```python
from build123d import *

# Parameters (mm, degrees)
F0_W          = 76.2
F0_H          = 38.1
F1_DEPTH      = 25.4
F2_W          = 69.85
F2_H          = 2.54
F3_DEPTH      = 38.101
F4_W          = 63.5
F4_H          = 25.4
F5_DEPTH      = 12.7
F6_W          = 6.35
F6_H          = 8.89
F7_DEPTH      = 6.35
F8_R          = 1.905
F9_DEPTH      = 6.35
F10_T1_DEPTH  = 76.2
F11_T1_DEPTH  = 17.78
F11_T3_DEPTH  = 55.88
F11_T5_DEPTH  = 7.62
F11_T7_DEPTH  = 7.62
F11_T10_ANGLE = 90.0000000017
F11_T12_ANGLE = 89.9999999998
F11_T14_ANGLE = 89.9999999979
F11_T16_ANGLE = 89.9999999998
F11_T18_ANGLE = 89.9999999998
F11_T20_ANGLE = 89.9999999998
F11_T22_ANGLE = 89.9999999979
F11_T24_ANGLE = 90.0000000017


# Not quite as in the source:
# - a fillet or chamfer that OpenCascade refuses, or shapes differently, is made with other operations: its cross-section is extruded or revolved along the edge and cut away or added


with BuildPart() as f1:
    # F0 (on Top) → F1 (new body)
    with BuildSketch(Plane.XY):
        with Locations((-11.0715073586, -8.5605031371)):
            Rectangle(F0_W, F0_H)
    extrude(amount=F1_DEPTH)

    # F2 (on face) → F3 (cut, through all)
    with BuildSketch(Plane.XZ.offset(27.6105031371)):
        with Locations((-11.0715073586, 3.81)):
            Rectangle(F2_W, F2_H)
    extrude(amount=-F3_DEPTH, mode=Mode.SUBTRACT)

    # F4 (on face) → F5 (cut)
    with BuildSketch(Plane.XY.offset(25.4)):
        with Locations((-11.0715073586, -8.5605031371)):
            Rectangle(F4_W, F4_H)
    extrude(amount=-F5_DEPTH, mode=Mode.SUBTRACT)

    # F6 (on face) → F7 (cut)
    with BuildSketch(Plane.XY.offset(25.4)):
        with Locations((23.8534926414, -8.5605031371)):
            Rectangle(F6_W, F6_H)
    extrude(amount=-F7_DEPTH, mode=Mode.SUBTRACT)

    # F8 (on face) → F9 (cut)
    with BuildSketch(Plane.XY.offset(25.4)):
        with Locations((-40.2815073586, 7.3144968629)):
            Circle(F8_R)
        with Locations((18.1384926414, 7.3144968629)):
            Circle(F8_R)
        with Locations((-40.2815073586, -24.4355031371)):
            Circle(F8_R)
        with Locations((18.1384926414, -24.4355031371)):
            Circle(F8_R)
    extrude(amount=-F9_DEPTH, mode=Mode.SUBTRACT)

    # F10: fillet of radius 10.16 on 4 edges, made by hand

    # F10_s2 → F10_t1 (cut)
    with BuildSketch(Plane.XY.offset(-25.4)):
        with BuildLine():
            ThreePointArc((-39.0115073586, -27.6105031371), (-46.1957122554, -24.634708034), (-49.1715073586, -17.4505031371))
            Line((-49.1715073586, -17.4505031371), (-49.1715073586, -27.6105031371))
            Line((-49.1715073586, -27.6105031371), (-39.0115073586, -27.6105031371))
        make_face()
        with BuildLine():
            ThreePointArc((27.0284926414, -17.4505031371), (24.0526975383, -24.634708034), (16.8684926414, -27.6105031371))
            Line((16.8684926414, -27.6105031371), (27.0284926414, -27.6105031371))
            Line((27.0284926414, -27.6105031371), (27.0284926414, -17.4505031371))
        make_face()
        with BuildLine():
            ThreePointArc((27.0284926414, 0.3294968629), (24.0526975383, 7.5137017597), (16.8684926414, 10.4894968629))
            Line((16.8684926414, 10.4894968629), (27.0284926414, 10.4894968629))
            Line((27.0284926414, 10.4894968629), (27.0284926414, 0.3294968629))
        make_face()
        with BuildLine():
            ThreePointArc((-39.0115073586, 10.4894968629), (-46.1957122554, 7.5137017597), (-49.1715073586, 0.3294968629))
            Line((-49.1715073586, 0.3294968629), (-49.1715073586, 10.4894968629))
            Line((-49.1715073586, 10.4894968629), (-39.0115073586, 10.4894968629))
        make_face()
    extrude(amount=F10_T1_DEPTH, mode=Mode.SUBTRACT)

    # F11: fillet of radius 1.27 on 17 edges, made by hand

    # F11_s2 → F11_t1 (cut)
    with BuildSketch(Plane.XZ.offset(-0.3294968629)):
        with BuildLine():
            ThreePointArc((-47.9015073586, 25.4), (-48.7995329707, 25.0280256121), (-49.1715073586, 24.13))
            Line((-49.1715073586, 24.13), (-49.1715073586, 25.4))
            Line((-49.1715073586, 25.4), (-47.9015073586, 25.4))
        make_face()
        with BuildLine():
            ThreePointArc((27.0284926414, 1.27), (26.6565182536, 0.3719743879), (25.7584926414, 0))
            Line((25.7584926414, 0), (27.0284926414, 0))
            Line((27.0284926414, 0), (27.0284926414, 1.27))
        make_face()
        with BuildLine():
            ThreePointArc((-47.9015073586, 0), (-48.7995329707, 0.3719743879), (-49.1715073586, 1.27))
            Line((-49.1715073586, 1.27), (-49.1715073586, 0))
            Line((-49.1715073586, 0), (-47.9015073586, 0))
        make_face()
    extrude(amount=F11_T1_DEPTH, mode=Mode.SUBTRACT)

    # F11_s4 → F11_t3 (cut)
    with BuildSketch(Plane.YZ.offset(-39.0115073586)):
        with BuildLine():
            ThreePointArc((9.2194968629, 0), (10.117522475, 0.3719743879), (10.4894968629, 1.27))
            Line((10.4894968629, 1.27), (10.4894968629, 0))
            Line((10.4894968629, 0), (9.2194968629, 0))
        make_face()
        with BuildLine():
            ThreePointArc((-26.3405031371, 0), (-27.2385287492, 0.3719743879), (-27.6105031371, 1.27))
            Line((-27.6105031371, 1.27), (-27.6105031371, 0))
            Line((-27.6105031371, 0), (-26.3405031371, 0))
        make_face()
        with BuildLine():
            ThreePointArc((9.2194968629, 25.4), (10.117522475, 25.0280256121), (10.4894968629, 24.13))
            Line((10.4894968629, 24.13), (10.4894968629, 25.4))
            Line((10.4894968629, 25.4), (9.2194968629, 25.4))
        make_face()
        with BuildLine():
            ThreePointArc((-26.3405031371, 25.4), (-27.2385287492, 25.0280256121), (-27.6105031371, 24.13))
            Line((-27.6105031371, 24.13), (-27.6105031371, 25.4))
            Line((-27.6105031371, 25.4), (-26.3405031371, 25.4))
        make_face()
    extrude(amount=F11_T3_DEPTH, mode=Mode.SUBTRACT)

    # F11_s6 → F11_t5 (cut)
    with BuildSketch(Plane.XZ.offset(-0.3294968629)):
        with BuildLine():
            ThreePointArc((27.0284926414, 24.13), (26.6565182536, 25.0280256121), (25.7584926414, 25.4))
            Line((25.7584926414, 25.4), (27.0284926414, 25.4))
            Line((27.0284926414, 25.4), (27.0284926414, 24.13))
        make_face()
    extrude(amount=F11_T5_DEPTH, mode=Mode.SUBTRACT)

    # F11_s8 → F11_t7 (cut)
    with BuildSketch(Plane.XZ.offset(9.8305031371)):
        with BuildLine():
            ThreePointArc((27.0284926414, 24.13), (26.6565182536, 25.0280256121), (25.7584926414, 25.4))
            Line((25.7584926414, 25.4), (27.0284926414, 25.4))
            Line((27.0284926414, 25.4), (27.0284926414, 24.13))
        make_face()
    extrude(amount=F11_T7_DEPTH, mode=Mode.SUBTRACT)

    # F11_s9 → F11_t10 (revolve, cut)
    with BuildSketch(Plane.XZ.offset(17.4505031373)):
        with BuildLine():
            ThreePointArc((25.7584926414, 0), (26.6565182535, 0.3719743879), (27.0284926414, 1.27))
            Line((27.0284926414, 1.27), (27.0284926414, 0))
            Line((27.0284926414, 0), (25.7584926414, 0))
        make_face()
    revolve(axis=Axis((16.8684926416, -17.4505031373, 0), (0, 0, -1)), revolution_arc=F11_T10_ANGLE, mode=Mode.SUBTRACT)

    # F11_s11 → F11_t12 (revolve, cut)
    with BuildSketch(Plane.YZ.offset(-39.0115073586)):
        with BuildLine():
            ThreePointArc((-26.3405031371, 0), (-27.2385287492, 0.3719743879), (-27.6105031371, 1.27))
            Line((-27.6105031371, 1.27), (-27.6105031371, 0))
            Line((-27.6105031371, 0), (-26.3405031371, 0))
        make_face()
    revolve(axis=Axis((-39.0115073586, -17.4505031371, 0), (0, 0, -1)), revolution_arc=F11_T12_ANGLE, mode=Mode.SUBTRACT)

    # F11_s13 → F11_t14 (revolve, cut)
    with BuildSketch(Plane.XZ.offset(-0.3294968627)):
        with BuildLine():
            ThreePointArc((-47.9015073586, 0), (-48.7995329707, 0.3719743879), (-49.1715073586, 1.27))
            Line((-49.1715073586, 1.27), (-49.1715073586, 0))
            Line((-49.1715073586, 0), (-47.9015073586, 0))
        make_face()
    revolve(axis=Axis((-39.0115073584, 0.3294968627, 0), (0, 0, -1)), revolution_arc=F11_T14_ANGLE, mode=Mode.SUBTRACT)

    # F11_s15 → F11_t16 (revolve, cut)
    with BuildSketch(Plane.YZ.offset(16.8684926414)):
        with BuildLine():
            ThreePointArc((9.2194968629, 0), (10.117522475, 0.3719743879), (10.4894968629, 1.27))
            Line((10.4894968629, 1.27), (10.4894968629, 0))
            Line((10.4894968629, 0), (9.2194968629, 0))
        make_face()
    revolve(axis=Axis((16.8684926414, 0.3294968629, 0), (0, 0, -1)), revolution_arc=F11_T16_ANGLE, mode=Mode.SUBTRACT)

    # F11_s17 → F11_t18 (revolve, cut)
    with BuildSketch(Plane.YZ.offset(16.8684926414)):
        with BuildLine():
            ThreePointArc((10.4894968629, 24.13), (10.117522475, 25.0280256121), (9.2194968629, 25.4))
            Line((9.2194968629, 25.4), (10.4894968629, 25.4))
            Line((10.4894968629, 25.4), (10.4894968629, 24.13))
        make_face()
    revolve(axis=Axis((16.8684926414, 0.3294968629, 25.4), (0, 0, -1)), revolution_arc=F11_T18_ANGLE, mode=Mode.SUBTRACT)

    # F11_s19 → F11_t20 (revolve, cut)
    with BuildSketch(Plane.YZ.offset(-39.0115073586)):
        with BuildLine():
            ThreePointArc((-26.3405031371, 25.4), (-27.2385287492, 25.0280256121), (-27.6105031371, 24.13))
            Line((-27.6105031371, 24.13), (-27.6105031371, 25.4))
            Line((-27.6105031371, 25.4), (-26.3405031371, 25.4))
        make_face()
    revolve(axis=Axis((-39.0115073586, -17.4505031371, 25.4), (0, 0, -1)), revolution_arc=F11_T20_ANGLE, mode=Mode.SUBTRACT)

    # F11_s21 → F11_t22 (revolve, cut)
    with BuildSketch(Plane.XZ.offset(-0.3294968627)):
        with BuildLine():
            ThreePointArc((-47.9015073586, 25.4), (-48.7995329707, 25.0280256121), (-49.1715073586, 24.13))
            Line((-49.1715073586, 24.13), (-49.1715073586, 25.4))
            Line((-49.1715073586, 25.4), (-47.9015073586, 25.4))
        make_face()
    revolve(axis=Axis((-39.0115073584, 0.3294968627, 25.4), (0, 0, -1)), revolution_arc=F11_T22_ANGLE, mode=Mode.SUBTRACT)

    # F11_s23 → F11_t24 (revolve, cut)
    with BuildSketch(Plane.XZ.offset(17.4505031373)):
        with BuildLine():
            ThreePointArc((25.7584926414, 25.4), (26.6565182535, 25.0280256121), (27.0284926414, 24.13))
            Line((27.0284926414, 24.13), (27.0284926414, 25.4))
            Line((27.0284926414, 25.4), (25.7584926414, 25.4))
        make_face()
    revolve(axis=Axis((16.8684926416, -17.4505031373, 25.4), (0, 0, -1)), revolution_arc=F11_T24_ANGLE, mode=Mode.SUBTRACT)


solid = f1.part
```
Could you check a few things on this model? Use its own coordinates, in mm. A direction names the side the tool comes from. Round coordinates to 2 decimals unless told otherwise and drop trailing zeros. Loops run counter-clockwise (first coordinate to the right, second up) from the corner with the lowest first, then second, coordinate; pieces in that order, holes last. Notation, with made-up numbers: (74.25, 57.5) - (121.25, 57.5) arc R31 ccw to (121.25, 81.5) - close; hole circle Ø10 at (-29.5, 5.25). An arc over 180 degrees is marked (long way). Answer as CSV lines item,"result".
1. I want a section at A-A on z = 3.5. List the corners of the cut face in (x, y) for me, then the cut area to 3 significant figures.
Filled in:
outline,"(-49.17, -17.45) arc R10.16 ccw to (-46, -24.83) - (-46, 7.71) arc R10.16 ccw to (-49.17, 0.33) - close; (23.85, -24.83) arc R10.16 ccw to (27.03, -17.45) - (27.03, 0.33) arc R10.16 ccw to (23.85, 7.71) - close"
area,"178 mm^2"
2. I want a section at D-D on z = 14.25. List the corners of the cut face in (x, y) for me, then the cut area to 3 significant figures.
Filled in:
outline,"(-49.17, -17.45) arc R10.16 ccw to (-39.01, -27.61) - (16.87, -27.61) arc R10.16 ccw to (27.03, -17.45) - (27.03, 0.33) arc R10.16 ccw to (16.87, 10.49) - (-39.01, 10.49) arc R10.16 ccw to (-49.17, 0.33) - close; hole (-42.82, -21.26) - (20.68, -21.26) - (20.68, 4.14) - (-42.82, 4.14) - close"
area,"1,200 mm^2"
3. Please list where these lines run through material, in increasing order: line 1 along Z through (x, y) = (-8, -17.5); line 2 along Y through (x, z) = (-25, 16.75); line 3 along X through (y, z) = (-11.5, 17). Write a range as [from, to].
Filled in:
line 1,"z = [0, 2.54], [5.08, 12.7]"
line 2,"y = [-27.61, -21.26], [4.14, 10.49]"
line 3,"x = [-49.17, -42.82], [20.68, 27.03]"
4. We'd pull the mould along X, two halves only. Please class faces 1 (the face through (-46.12, 7.59, 12.54)), 2 (the face through (23.853, -9, 4)), 3 (the face through (24, -8, 19.05)): +X half, -X half, draft (parallel to the pull), parting line (faces both ways), or undercut.
Filled in:
face 1,"-X half"
face 2,"undercut"
face 3,"draft"
5. On a 3-axis mill with a long thin cutter (end or side, diameter ignored), from which of +Z, -Z, +X, -X, +Y, -Y can I reach the whole of each face in a straight line? I mean faces 4 (the face through (-40, -24, 19.05)), 5 (the face through (27.028, -9, 13)), 6 (the face through (24, -13.006, 22)), 7 (the face through (-45.997, -9, 4)), 8 (the face through (-11, -27.611, 14)). Say none if no direction works.
Filled in:
face 4,"+Z"
face 5,"+Z, -Z, +X, +Y, -Y"
face 6,"+Z, +X"
face 7,"+Y, -Y"
face 8,"+Z, -Z, +X, -X, -Y"
6. I want a section at C-C on y = -11. List the corners of the cut face in (x, z) for me, then the cut area to 3 significant figures.
Filled in:
outline,"(-49.17, 1.27) arc R1.27 ccw to (-47.9, 0) - (25.76, 0) arc R1.27 ccw to (27.03, 1.27) - (27.03, 19.05) - (20.68, 19.05) - (20.68, 12.7) - (-42.82, 12.7) - (-42.82, 25.4) - (-47.9, 25.4) arc R1.27 ccw to (-49.17, 24.13) - close; hole (-46, 2.54) - (23.85, 2.54) - (23.85, 5.08) - (-46, 5.08) - close"
area,"910 mm^2"
7. For pin 1 Ø10 at (x, y) = (10, -6) entering from +Z; pin 2 Ø3 at (x, y) = (23, -7) entering from +Z; pin 3 Ø3 at (y, z) = (-20.5, 12.5) entering from -X, each with a flat end and sliding along its axis, tell me the tip position at first contact or that it passes through.
Filled in:
pin 1,"stops at z = 12.7"
pin 2,"stops at z = 19.05"
pin 3,"stops at x = -49.05"
8. I want a section at B-B on x = 2.5. List the corners of the cut face in (y, z) for me, then the cut area to 3 significant figures.
Filled in:
outline,"(-27.61, 1.27) arc R1.27 ccw to (-26.34, 0) - (9.22, 0) arc R1.27 ccw to (10.49, 1.27) - (10.49, 2.54) - (-27.61, 2.54) - close; (-27.61, 5.08) - (10.49, 5.08) - (10.49, 24.13) arc R1.27 ccw to (9.22, 25.4) - (4.14, 25.4) - (4.14, 12.7) - (-21.26, 12.7) - (-21.26, 25.4) - (-26.34, 25.4) arc R1.27 ccw to (-27.61, 24.13) - close"
area,"547 mm^2"
